```python
from build123d import *

# Parameters (mm, degrees)
FILLET1_R          = 1.016
SKETCH5_R          = 3.556
CUT_EXTRUDE4_DEPTH = 2.701148395
SKETCH9_W          = 105.570120157
SKETCH9_H          = 128.790829306
CUT_EXTRUDE5_DEPTH = 1.27


with BuildPart() as part:
    # Sketch1 → Revolve1 (revolve)
    with BuildSketch(Plane.XY, mode=Mode.PRIVATE) as revolve1_sk:
        Polygon((-0.172820682, 49.639122622), (-0.172820682, 0.012009488), (-0.172820682, -2.194330865), (31.577179318, -2.194330865), (31.577179318, 0.506817529), (16.121405897, 0.506817529), (16.121405897, 2.63143161), (3.002179318, 2.63143161), (3.002179318, 47.08143161), (3.46467558, 47.08143161), (3.503063095, 49.639122622), align=None)
    revolve(revolve1_sk.sketch.rotate(Axis((-0.172820682, 49.639122622, 0), (0, -1, 0)), 90), axis=Axis((-0.172820682, 49.639122622, 0), (0, -1, 0)))

    # Fillet1
    fillet1_edges = [part.edges().sort_by_distance(p)[0] for p in [
        (-0.172820682, 0.506817529, -16.294226579),
        (-0.172820682, 2.63143161, -16.294226579),
    ]]
    fillet(fillet1_edges, radius=FILLET1_R)

    # Sketch5 → Cut-Extrude4 (cut)
    with BuildSketch(Plane(origin=(0, 0.506817529, 0), x_dir=(1, 0, 0), z_dir=(0, 1, 0))):
        with Locations(Location((-23.064919044, 6.522820682, 0), (0, 0, 270))):
            Circle(SKETCH5_R)
        with Locations(Location((6.522820682, 23.064919044, 0), (0, 0, 270))):
            Circle(SKETCH5_R)
        with Locations(Location((23.064919044, -6.522820682, 0), (0, 0, 270))):
            Circle(SKETCH5_R)
        with Locations(Location((-6.522820682, -23.064919044, 0), (0, 0, 270))):
            Circle(SKETCH5_R)
    extrude(amount=-CUT_EXTRUDE4_DEPTH, mode=Mode.SUBTRACT)

    # Sketch9 → Cut-Extrude5 (cut, symmetric)
    with BuildSketch(Plane.XY):
        with Locations((-17.353763652, 67.026846263)):
            Rectangle(SKETCH9_W, SKETCH9_H)
    extrude(amount=CUT_EXTRUDE5_DEPTH, both=True, mode=Mode.SUBTRACT)


solid = part.part
```
Geometry: final body of the model. Coordinates: model frame, mm. A direction names the side the tool comes from. Round coordinates to 2 decimals unless told otherwise and drop trailing zeros. Loops run counter-clockwise (first coordinate to the right, second up) from the corner with the lowest first, then second, coordinate; pieces in that order, holes last. Notation, with made-up numbers: (26.25, 75) -> (62.25, 75) arc R23 cw to (62.25, 86) -> close; hole circle Ø8 at (62, 59.5). An arc over 180 degrees is marked (long way). Use one line per item in the form item = value. Start each with the question number.
1) Section B-B on z = 0. Output: boundary loops of the cut face in (x, y).
2) Access query for faces 1 (the flat face through (0, 26, -1.27)), 2 (the cylindrical face through (-0.224, 25.168, -3.175)). Directions: +Z, -Z, +X, -X, +Y, -Y. A direction counts if a zero-diameter tool reaches every point of the face in a straight line with its end or side. Return the directions, or none.
3) First-contact query: P1, Ø6, axis at x = 6, y = 4.5, coming from the -Z side; P2, Ø3.5, axis at x = -1, y = 18, coming from the +Z side (3 decimals); P3, Ø2, axis at x = -0.5, y = 18, coming from the -Z side (3 decimals). Flat tips, straight axial feed; report the tip coordinate or a pass-through.
4) Section D-D on x = 24.5. Output: boundary loops of the cut face in (y, z), then the cut area to 3 significant figures.
5) Section C-C on y = 18.5. Output: boundary loops of the cut face in (x, z) (3 decimals), then the cut area to 3 significant figures.
6) Draft query along Y for faces 3 (the flat face through (0, 49.639, 2)), 4 (the conical face through (-0.11, 48.378, 3.656)), 5 (the cylindrical face through (-6.366, -0.825, 19.512)). Return one class per face: released by +Y, released by -Y, zero draft, split by the parting line, or undercut.
7) Line query: L1, parallel to Z at x = -0.5, y = 47; L2, parallel to Y at x = 22, z = 1.5; L3, parallel to Z at x = 1, y = 17. Output: solid intervals per line, ascending.
8) Section A-A on x = -24.5. Output: boundary loops of the cut face in (y, z).
Response:
q1.outline = (-31.92, -2.19) -> (31.58, -2.19) -> (31.58, 0.51) -> (17.14, 0.51) arc R1.02 cw to (16.12, 1.52) -> (16.12, 1.62) arc R1.02 ccw to (15.11, 2.63) -> (-15.45, 2.63) arc R1.02 ccw to (-16.47, 1.62) -> (-16.47, 1.52) arc R1.02 cw to (-17.48, 0.51) -> (-31.92, 0.51) -> close
q2.face_1 = +X, -X, +Y
q2.face_2 = -Z
q3.P1 = -15.58
q3.P2 = 3.175
q3.P3 = -3.175
q4.outline = (-2.19, -19.98) -> (0.51, -19.98) -> (0.51, 3.27) -> (-2.19, 3.27) -> close; (-2.19, 9.78) -> (0.51, 9.78) -> (0.51, 19.98) -> (-2.19, 19.98) -> close
q4.area = 90.4 mm^2
q5.outline = (-3.083, -1.27) arc R3.175 ccw to (2.737, -1.27) -> close; (-3.083, 1.27) -> (2.737, 1.27) arc R3.175 ccw to start
q5.area = 16.0 mm^2
q6.face_3 = released by +Y
q6.face_4 = undercut
q6.face_5 = zero draft
q7.L1 = -3.16 to -1.27, 1.27 to 3.16
q7.L2 = -2.19 to 0.51
q7.L3 = -2.95 to -1.27, 1.27 to 2.95
q8.outline = (-2.19, -20.4) -> (0.51, -20.4) -> (0.51, -9.78) -> (-2.19, -9.78) -> close; (-2.19, -3.27) -> (0.51, -3.27) -> (0.51, 20.4) -> (-2.19, 20.4) -> close
